The listing builds one solid part. Answer for the finished solid, in the listing's coordinates (mm). A direction names the side the tool comes from. Give positions to 0.01 mm unless a question says otherwise; leave off trailing zeros. Write each loop counter-clockwise with the first axis right and the second up, starting at its lowest first coordinate (ties: lowest second). Pieces come first, ordered by that corner, then holes. Notation, with made-up numbers: (64, 85) - (70, 85) arc R12 cw to (70, 99) - close; hole circle Ø9 at (-1, 24). An arc over 180 degrees is marked (long way). Return JSON: item names as keys, results as strings.
Autodesk Inventor part; units mm, degrees
ref_plane "YZ Plane" through (0, 0, 0) normal (1, 0, 0) x (0, 1, 0)
ref_plane "XZ Plane" through (0, 0, 0) normal (0, 1, 0) x (-1, 0, 0)
ref_plane "XY Plane" through (0, 0, 0) normal (0, 0, 1) x (1, 0, 0)
sketch "Skizze1" plane through (0, 0, 0) normal (0, 0, 1) x (1, 0, 0)
  line L0 (-8.4, 0) -> (8.4, 0)
  line L1 (0, -2) -> (0, 12)
  line L2 (6, 10) -> (6, 0)
  line L3 (6, 0) -> (-6, 0)
  line L4 (-6, 0) -> (-6, 10)
  line L5 (4.5, 10) -> (4.5, 2)
  line L6 (4.5, 2) -> (-4.5, 2)
  line L7 (-4.5, 2) -> (-4.5, 10)
  line L8 (-6, 10) -> (-4.5, 10)
  line L9 (4.5, 10) -> (6, 10)
  point P0 (0, 0)
  dimension "d0" = 2
  dimension "d2" = 9
  dimension "d3" = 1.5
  dimension "d4" = 10
extrude "Extrusion1" add sketch "Skizze1" along normal blind 40
sketch "Skizze2" plane through (-6, 0, 0) normal (0, -1, 0) x (1, 0, 0)
  line L0 (0, 0) -> (12, 0)
  line L1 (12, 0) -> (12, 40)
  point P0 (6, 0)
  point P1 (6, 2.5)
  dimension "d7" = 2.5
  dimension "d8" = 6
hole "Bohrung1" at (0, 0, 2.5) direction (0, 1, 0) diameter 2.4 end through all countersink diameter 4.5 countersink angle 90
sketch "Skizze3" plane through (-6, 0, 0) normal (-1, 0, 0) x (0, 0, 1)
  line L0 (0, 0) -> (40, 0)
  line L1 (40, 10) -> (40, 0)
  line L2 (35, 5) -> (28, 5) construction
  line L3 (35, 2.5) -> (28, 2.5)
  line L4 (28, 7.5) -> (35, 7.5)
  arc A0 (35, 2.5) -> (35, 7.5) centre (35, 5) ccw
  arc A1 (28, 7.5) -> (28, 2.5) centre (28, 5) ccw
  point P0 (31.5, 5)
  dimension "d16" = 5
  dimension "d17" = 5
  dimension "d18" = 5
  dimension "d19" = 7
extrude "Extrusion2" cut sketch "Skizze3" against normal through all
pattern_linear "Rechteckige Anordnung1" count 2 spacing 15 along (0, 0, -1) of "Extrusion2"
fillet "Rundung1" radius 5 2 edges at (5.25, 10, 40) (-5.25, 10, 40)
properties part number "13_1087_001" material "Kupfer"
Item 1: A cutting plane is placed at A-A on x = 0. Determine the outline of the cut face in (y, z).
Answer below:
{"outline": "(0, 0) - (2, 0) - (2, 1.3) - (1.05, 1.3) - (0, 0.25) - close; (0, 4.75) - (1.05, 3.7) - (2, 3.7) - (2, 40) - (0, 40) - close"}
Item 2: A cutting plane is placed at D-D on y = 3.25. Determine the outline of the cut face in (x, z).
Answer below:
{"outline": "(-6, 0) - (-4.5, 0) - (-4.5, 11.21) - (-6, 11.21) - close; (-6, 21.79) - (-4.5, 21.79) - (-4.5, 26.21) - (-6, 26.21) - close; (-6, 36.79) - (-4.5, 36.79) - (-4.5, 40) - (-6, 40) - close; (4.5, 0) - (6, 0) - (6, 11.21) - (4.5, 11.21) - close; (4.5, 21.79) - (6, 21.79) - (6, 26.21) - (4.5, 26.21) - close; (4.5, 36.79) - (6, 36.79) - (6, 40) - (4.5, 40) - close"}
Item 3: The mould has two halves that part along Z. Classify faces 3 (the face through (0, 0, 20)), 4 (the face through (-5, 9, 38)), 5 (the face through (-5.3, 4.9, 22.5)): +Z half, -Z half, draft (parallel to the pull), parting line (faces both ways), or undercut.
Answer below:
{"face 3": "draft", "face 4": "+Z half", "face 5": "undercut"}
Item 4: For faces 1 (the face through (-0.1, 1.7, 0)), 2 (the face through (-5.3, 5.1, 10.5)), determine the directions among +Z, -Z, +X, -X, +Y, -Y from which every point of the face is accessible in a straight line to the end or side of a thin tool.
Answer below:
{"face 1": "-Z, +X, -X, +Y, -Y", "face 2": "+X, -X"}
Item 5: A flat-ended cylindrical pin translates along its axis: P1, Ø3, axis at x = 0, z = 2.5, coming from the +Y side. Find the tip coordinate at first contact, or state that the pin passes through.
Answer below:
{"P1": "stops at y = 2"}
Item 6: Consider L1, parallel to Z at x = 0, y = 1.8; L2, parallel to Y at x = -4.75, z = 32; L3, parallel to Z at x = 5.75, y = 7. Determine where each line is inside the solid, lowest interval first.
Answer below:
{"L1": "z = 0 to 1.3, 3.7 to 40", "L2": "y = 0 to 2.5, 7.5 to 10", "L3": "z = 0 to 11.5, 21.5 to 26.5, 36.5 to 39.58"}
Item 7: A cutting plane is placed at B-B on z = 2.5. Determine the outline of the cut face in (x, y), then the cut area to 3 significant figures.
Answer below:
{"outline": "(-6, 0) - (-2.25, 0) - (-1.2, 1.05) - (-1.2, 2) - (-4.5, 2) - (-4.5, 10) - (-6, 10) - close; (1.2, 1.05) - (2.25, 0) - (6, 0) - (6, 10) - (4.5, 10) - (4.5, 2) - (1.2, 2) - close", "area": "42.1 mm²"}
Item 8: A cutting plane is placed at C-C on z = 32. Determine the outline of the cut face in (x, y), then the cut area to 3 significant figures.
Answer below:
{"outline": "(-6, 0) - (6, 0) - (6, 2.5) - (4.5, 2.5) - (4.5, 2) - (-4.5, 2) - (-4.5, 2.5) - (-6, 2.5) - close; (-6, 7.5) - (-4.5, 7.5) - (-4.5, 10) - (-6, 10) - close; (4.5, 7.5) - (6, 7.5) - (6, 10) - (4.5, 10) - close", "area": "33.0 mm²"}
